Can you work these out from the model? Positions are in its coordinate system, mm. Round coordinates to 2 decimals unless told otherwise and drop trailing zeros. Order: outer loops, then holes, each group sorted by start corner. A loop starts at its lowest first (then second) coordinate and runs counter-clockwise, first axis right, second up. Notation, with made-up numbers: (13.5, -16.75) -> (41.5, -16.75) arc R27 cw to (41.5, 17.25) -> close; hole circle Ø3 at (-31, 35.25). An arc over 180 degrees is marked (long way). One line per item, written item: value.
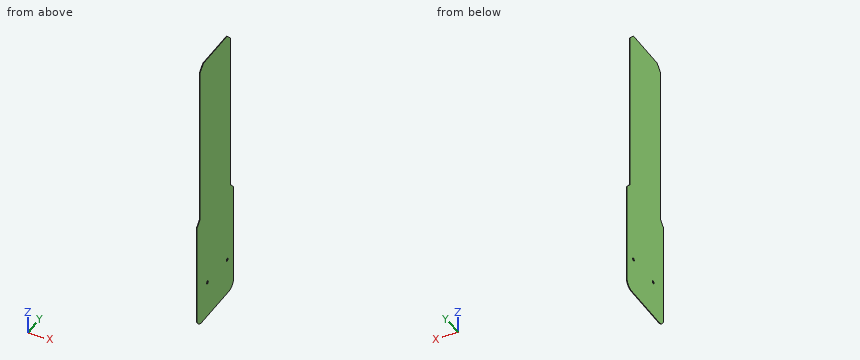
```python
from build123d import *

# Parameters (mm, degrees)
SKETCH2_W           = 22.42
SKETCH2_H           = 92
BOSS_EXTRUDE2_DEPTH = 0.2
FILLET4_R           = 3
FILLET7_R           = 3
SKETCH4_W           = 2
SKETCH4_H           = 54.51
CUT_EXTRUDE1_DEPTH  = 0.2
SKETCH5_W           = 2
SKETCH5_H           = 54.51
CUT_EXTRUDE2_DEPTH  = 0.2
CUT_EXTRUDE3_DEPTH  = 0.2
CUT_EXTRUDE4_DEPTH  = 0.2
CUT_EXTRUDE7_DEPTH  = 0.2
CUT_EXTRUDE8_DEPTH  = 0.2
SKETCH13_R          = 0.5
CUT_EXTRUDE12_DEPTH = 10
SKETCH15_R          = 0.5
CUT_EXTRUDE13_DEPTH = 0.2


with BuildPart() as part:
    # Sketch2 → Boss-Extrude2 (new body)
    with BuildSketch(Plane(origin=(0, 0, 0), x_dir=(0, 1, 0), z_dir=(-1, 0, 0))):
        with Locations((-43.813076923, -17.338461538)):
            Rectangle(SKETCH2_W, SKETCH2_H)
    extrude(amount=BOSS_EXTRUDE2_DEPTH)

    # Fillet4
    fillet4_edges = [part.edges().sort_by_distance(p)[0] for p in [
        (-0.1, -55.023076923, -28.661538462),
    ]]
    fillet(fillet4_edges, radius=FILLET4_R)

    # Fillet7
    fillet7_edges = [part.edges().sort_by_distance(p)[0] for p in [
        (-0.1, -32.603076923, -28.661538462),
    ]]
    fillet(fillet7_edges, radius=FILLET7_R)

    # Sketch4 → Cut-Extrude1 (cut)
    with BuildSketch(Plane(origin=(-0.2, 0, 0), x_dir=(0, 1, 0), z_dir=(-1, 0, 0))):
        with Locations((-54.023076923, -36.083461538)):
            Rectangle(SKETCH4_W, SKETCH4_H)
    extrude(amount=-CUT_EXTRUDE1_DEPTH, mode=Mode.SUBTRACT)

    # Sketch5 → Cut-Extrude2 (cut)
    with BuildSketch(Plane(origin=(-0.2, 0, 0), x_dir=(0, 1, 0), z_dir=(-1, 0, 0))):
        with Locations((-33.603076923, -36.083461538)):
            Rectangle(SKETCH5_W, SKETCH5_H)
    extrude(amount=-CUT_EXTRUDE2_DEPTH, mode=Mode.SUBTRACT)

    # Sketch6 → Cut-Extrude3 (cut)
    with BuildSketch(Plane(origin=(-0.2, 0, 0), x_dir=(0, 1, 0), z_dir=(-1, 0, 0))):
        Polygon((-53.023076923, -63.338461538), (-53.023076923, -61.338461538), (-51.023076923, -63.338461538), align=None)
    extrude(amount=-CUT_EXTRUDE3_DEPTH, mode=Mode.SUBTRACT)

    # Sketch7 → Cut-Extrude4 (cut)
    with BuildSketch(Plane(origin=(-0.2, 0, 0), x_dir=(0, 1, 0), z_dir=(-1, 0, 0))):
        Polygon((-34.603076923, -63.338461538), (-34.603076923, -61.338461538), (-36.603076923, -63.338461538), align=None)
    extrude(amount=-CUT_EXTRUDE4_DEPTH, mode=Mode.SUBTRACT)

    # Sketch8 → Cut-Extrude7 (cut)
    with BuildSketch(Plane(origin=(-0.2, 0, 0), x_dir=(0, 1, 0), z_dir=(-1, 0, 0))):
        Polygon((-53.023076923, -8.828461538), (-55.023076923, -8.828461538), (-55.023076923, -6.828461538), align=None)
    extrude(amount=-CUT_EXTRUDE7_DEPTH, mode=Mode.SUBTRACT)

    # Sketch9 → Cut-Extrude8 (cut)
    with BuildSketch(Plane(origin=(-0.2, 0, 0), x_dir=(0, 1, 0), z_dir=(-1, 0, 0))):
        Polygon((-34.603076923, -8.828461538), (-32.603076923, -8.828461538), (-32.603076923, -6.828461538), align=None)
    extrude(amount=-CUT_EXTRUDE8_DEPTH, mode=Mode.SUBTRACT)

    # Sketch13 → Cut-Extrude12 (cut)
    with BuildSketch(Plane(origin=(-0.2, 0, 0), x_dir=(0, 1, 0), z_dir=(-1, 0, 0))):
        with Locations(Location((-48.603076923, 16.661538462, 0), (0, 0, 180))):
            Circle(SKETCH13_R)
    extrude(amount=-CUT_EXTRUDE12_DEPTH, mode=Mode.SUBTRACT)

    # Sketch15 → Cut-Extrude13 (cut)
    with BuildSketch(Plane(origin=(-0.2, 0, 0), x_dir=(0, 1, 0), z_dir=(-1, 0, 0))):
        with Locations(Location((-36.603076923, 16.661538462, 0), (0, 0, 180))):
            Circle(SKETCH15_R)
    extrude(amount=-CUT_EXTRUDE13_DEPTH, mode=Mode.SUBTRACT)


solid = part.part
```
Q1. I want a section at B-B on z = 37. List the corners of the cut face in (x, y) for me, plus the area to 3 significant figures.
Answers below:
outline: (-0.2, -53.02) -> (0, -53.02) -> (0, -34.6) -> (-0.2, -34.6) -> close
area: 3.68 mm^2
Q2. I want a section at A-A on x = -0.05. List the corners of the cut face in (y, z) for me.
Answers below:
outline: (-55.02, -25.66) arc R3 ccw to (-52.02, -28.66) -> (-35.6, -28.66) arc R3 ccw to (-32.6, -25.66) -> (-32.6, 6.83) -> (-34.6, 8.83) -> (-34.6, 61.34) -> (-36.6, 63.34) -> (-51.02, 63.34) -> (-53.02, 61.34) -> (-53.02, 8.83) -> (-55.02, 6.83) -> close; hole circle Ø1 at (-48.6, -16.66); hole circle Ø1 at (-36.6, -16.66)
Q3. Please list where these lines run through material, in increasing order: line 1 along Y through (x, z) = (-0.15, 10.5); line 2 along Z through (x, y) = (-0.1, -36); line 3 along Z through (x, y) = (-0.1, -35).
Answers below:
line 1: -53.02 to -34.6
line 2: -28.66 to 62.74
line 3: -28.6 to 61.74
